Input: dimensioned drawing with shaded views. Units: mm. Origin: part minimum x, y, z. Round coordinates to 2 decimals unless told otherwise and drop trailing zeros. Loops run counter-clockwise (first coordinate to the right, second up) from the corner with the lowest first, then second, coordinate; pieces in that order, holes last. Notation, with made-up numbers: M -35.75,2 L -17.75,2 A21 cw -17.75,40 Z; hole C -10.5,3 d4. An arc over 180 degrees is marked long. Return JSON: item names as keys, results as strings.
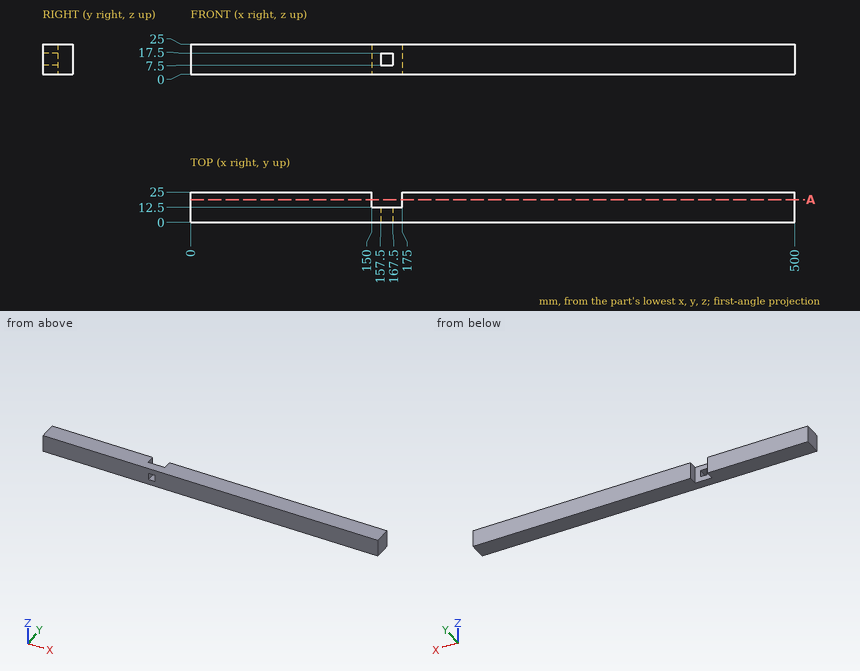
Q1. Section query A-A (y = 18.75). Output: boundary loops of the cut face in (x, z), plus the area to 3 significant figures.
Determined:
{"outline": "M 0,0 L 150,0 L 150,25 L 0,25 Z; M 175,0 L 500,0 L 500,25 L 175,25 Z", "area": "11,900 mm^2"}
Q2. Pin query (flat end, axial travel): pin 1 (12.5 mm diameter, centred on x = 163.5, z = 12, fed in from +Y). Return the tip coordinate at first contact, or that it passes through.
Determined:
{"pin 1": "stops at y = 12.5"}
Q3. Material intervals for L1, parallel to X at y = 13, z = 16; L2, parallel to X at y = 7.75, z = 8.25; L3, parallel to Z at x = 160.5, y = 11.25, sorted ascending.
Determined:
{"L1": "x = 0 to 150, 175 to 500", "L2": "x = 0 to 157.5, 167.5 to 500", "L3": "z = 0 to 7.5, 17.5 to 25"}
